Read the model definition and answer for the solid it produces. Units are mm, in the model's axes. A direction names the side the tool comes from. Coordinates: 2 decimals unless noted, no trailing zeros. Order: outer loops, then holes, each group sorted by start corner. A loop starts at its lowest first (then second) coordinate and runs counter-clockwise, first axis right, second up. Notation, with made-up numbers: (38.5, -18) - (67.5, -18) arc R22 cw to (67.5, -12) - close; hole circle Ø3 at (2, 29.5). An arc over 180 degrees is marked (long way). Write item = value, one per line.
from build123d import *

# Parameters (mm, degrees)
SKETCH1_W               = 60
SKETCH1_H               = 45
BOSS_EXTRUDE1_DEPTH     = 2
SKETCH2_W               = 2
SKETCH2_H               = 45
BOSS_EXTRUDE2_DEPTH     = 20
CUT_EXTRUDE1_DEPTH      = 68.75138375
CUT_EXTRUDE1_DEPTH_BACK = 68.75138375
SKETCH3_R               = 2
SKETCH3_R_2             = 4.5
SKETCH3_R_3             = 2.5


with BuildPart() as part:
    # Sketch1 → Boss-Extrude1 (new body)
    with BuildSketch(Plane(origin=(0, 0, 0), x_dir=(1, 0, 0), z_dir=(0, 1, 0))):
        Rectangle(SKETCH1_W, SKETCH1_H)
    extrude(amount=BOSS_EXTRUDE1_DEPTH)

    # Sketch2 → Boss-Extrude2 (add)
    with BuildSketch(Plane(origin=(0, 2, 0), x_dir=(1, 0, 0), z_dir=(0, 1, 0))):
        with Locations((-29, 0)):
            Rectangle(SKETCH2_W, SKETCH2_H)
        with Locations((29, 0)):
            Rectangle(SKETCH2_W, SKETCH2_H)
    extrude(amount=BOSS_EXTRUDE2_DEPTH)

    # Sketch3 → Cut-Extrude1 (cut, two sides: drawn at the far end of the back side and taken through both)
    with BuildSketch(Plane(origin=(30, 0, 0), x_dir=(0, 0, -1), z_dir=(1, 0, 0)).offset(-CUT_EXTRUDE1_DEPTH_BACK)):
        with Locations((-17.5, 8)):
            Circle(SKETCH3_R)
        with Locations((17.5, 8)):
            Circle(SKETCH3_R)
        with Locations((0, 16)):
            Circle(SKETCH3_R_2)
        with Locations((17.5, 16)):
            Circle(SKETCH3_R_3)
        with Locations((-17.5, 16)):
            Circle(SKETCH3_R_3)
    extrude(amount=CUT_EXTRUDE1_DEPTH + CUT_EXTRUDE1_DEPTH_BACK, mode=Mode.SUBTRACT)


solid = part.part
1) For faces 4 (the face through (-29, 22, 0)), 5 (the face through (0, 2, 0)), determine the directions among +Z, -Z, +X, -X, +Y, -Y from which every point of the face is accessible in a straight line to the end or side of a thin tool.
Returned:
face_4 = +Z, -Z, +X, -X, +Y
face_5 = +Z, -Z, +Y
2) Determine the mould class of faces 1 (the face through (30, 11, 0)), 2 (the face through (28, 10, 0)), 3 (the face through (29, 16, 20)) for opening direction X: pulls with the +X half, pulls with the -X half, needs draft (parallel to the pull), parting line crosses it, or undercut.
Returned:
face_1 = pulls with the +X half
face_2 = undercut
face_3 = needs draft
3) The part is cut by section A-A (y = 8). Determine the outline of the cut face in (x, z).
Returned:
outline = (-30, -22.5) - (-28, -22.5) - (-28, -19.5) - (-30, -19.5) - close; (-30, -15.5) - (-28, -15.5) - (-28, 15.5) - (-30, 15.5) - close; (-30, 19.5) - (-28, 19.5) - (-28, 22.5) - (-30, 22.5) - close; (28, -22.5) - (30, -22.5) - (30, -19.5) - (28, -19.5) - close; (28, -15.5) - (30, -15.5) - (30, 15.5) - (28, 15.5) - close; (28, 19.5) - (30, 19.5) - (30, 22.5) - (28, 22.5) - close
4) The part is cut by section D-D (z = 1.5). Determine the outline of the cut face in (x, y).
Returned:
outline = (-30, 0) - (30, 0) - (30, 11.76) - (28, 11.76) - (28, 2) - (-28, 2) - (-28, 11.76) - (-30, 11.76) - close; (-30, 20.24) - (-28, 20.24) - (-28, 22) - (-30, 22) - close; (28, 20.24) - (30, 20.24) - (30, 22) - (28, 22) - close
5) Straight lines are drawn through the part: line 1 along Z through (x, y) = (28.5, 8); line 2 along Y through (x, z) = (29.5, -17.5); line 3 along Z through (x, y) = (-29.25, 16). For each, find the intervals that lie inside material, in ascending order. Write a range as from..to.
Returned:
line_1 = -22.5..-19.5, -15.5..15.5, 19.5..22.5
line_2 = 0..6, 10..13.5, 18.5..22
line_3 = -22.5..-20, -15..-4.5, 4.5..15, 20..22.5
6) The part is cut by section C-C (z = 17.5). Determine the outline of the cut face in (x, y), and give its area (3 significant figures).
Returned:
outline = (-30, 0) - (30, 0) - (30, 6) - (28, 6) - (28, 2) - (-28, 2) - (-28, 6) - (-30, 6) - close; (-30, 10) - (-28, 10) - (-28, 13.5) - (-30, 13.5) - close; (-30, 18.5) - (-28, 18.5) - (-28, 22) - (-30, 22) - close; (28, 10) - (30, 10) - (30, 13.5) - (28, 13.5) - close; (28, 18.5) - (30, 18.5) - (30, 22) - (28, 22) - close
area = 164 mm^2
7) Flat-ended cylindrical pins translate along their axes: pin 1 Ø1.5 at (x, y) = (-12.5, 2.5) entering from -Z; pin 2 Ø3.5 at (y, z) = (8, -17.5) entering from -X; pin 3 Ø4 at (x, z) = (12.5, -4.5) entering from +Y. Find the tip coordinate at first contact, or state that the pin passes through.
Returned:
pin_1 = -22.5
pin_2 = through
pin_3 = 2
8) The part is cut by section B-B (y = 16). Count the separate pieces of the cut face and the enclosed holes in it, and give its area (3 significant figures).
Returned:
separate_pieces = 8
enclosed_holes = 0
area = 104 mm^2
